from build123d import *

# Parameters (mm, degrees)
BOSS_EXTRUDE1_DEPTH = 24.14


with BuildPart() as part:
    # Sketch3 → Boss-Extrude1 (new body)
    with BuildSketch(Plane.XY):
        with BuildLine():
            Line((6.42, 0), (393.58, 0))
            ThreePointArc((393.58, 0), (402.030182258, -6.090546773), (405.136, 3.852))
            Line((405.136, 3.852), (794.864, 296.148))
            ThreePointArc((794.864, 296.148), (806.090546773, 302.030182258), (793.58, 300))
            Line((793.58, 300), (-393.58, 300))
            ThreePointArc((-393.58, 300), (-406.090546773, 302.030182258), (-394.864, 296.148))
            Line((-394.864, 296.148), (-5.136, 3.852))
            ThreePointArc((-5.136, 3.852), (-2.030182258, -6.090546773), (6.42, 0))
        make_face()
        Polygon((64.373333333, 24.14), (719.533333333, 269.825), (391.953333333, 24.14), align=None, mode=Mode.SUBTRACT)
        Polygon((-327.58, 275.86), (3.90530551, 27.246020868), (666.875916529, 275.86), align=None, mode=Mode.SUBTRACT)
    extrude(amount=BOSS_EXTRUDE1_DEPTH)


solid = part.part
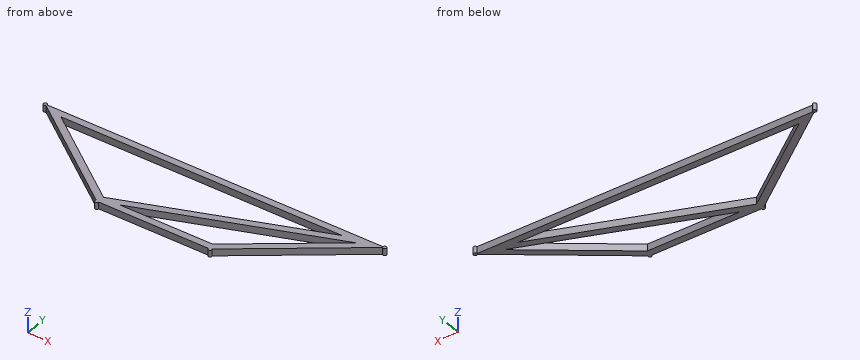
Could you check a few things on this model? Use its own coordinates, in mm. Coordinates: 2 decimals unless noted, no trailing zeros. Order: outer loops, then holes, each group sorted by start corner. A loop starts at its lowest first (then second) coordinate and runs counter-clockwise, first axis right, second up. Notation, with made-up numbers: (40.5, -17.5) - (96.5, -17.5) arc R19 ccw to (96.5, 11.5) - close; hole circle Ø7 at (-19, 65.5). An arc over 180 degrees is marked (long way). Answer in a Markdown table with one row per item. Add a question column.
(1) If we section it at D-D, the plane x = 180.5: Please give me the cut outline in (y, z).
(2) If we section it at B-B, the plane x = -73: Please give me the cut outline in (y, z) (3 decimals), then the cut area to 3 significant figures.
(3) Will these pins go through, and if not, where does the flat tip stop? pin 1 (12 mm diameter, centred on x = 234, z = 16, fed in from -Y); pin 2 (10 mm diameter, centred on x = -86.5, y = 81.5, fed in from -Z); pin 3 (8 mm diameter, centred on y = 264, z = 3, fed in from +X); pin 4 (3 mm diameter, centred on y = 116.5, z = 20, fed in from +X).
(4) If we section it at A-A, the plane z = 15.25: Please give me the cut outline in (x, y) (3 decimals).
(5) If we section it at C-C, the plane y = 206.5: Please give me the cut outline in (x, z).
(6) I need wall thicknesses on L1, parallel to Y at x = 152.5, z = 4.25; L2, parallel to Y at x = 194.5, z = 15.25; L3, parallel to Y at x = -159, z = 8.25 (3 decimals). Which ranges of each line are inside material? Lowest first, please.
Results are:
| question | item | result |
|---|---|---|
| 1 | outline | (0, 0) - (24.14, 0) - (24.14, 24.14) - (0, 24.14) - close; (67.69, 0) - (93.47, 0) - (93.47, 24.14) - (67.69, 24.14) - close; (275.86, 0) - (300, 0) - (300, 24.14) - (275.86, 24.14) - close |
| 2 | outline | (54.75, 0) - (84.925, 0) - (84.925, 24.14) - (54.75, 24.14) - close; (275.86, 0) - (300, 0) - (300, 24.14) - (275.86, 24.14) - close |
| 2 | area | 1,310 mm2 |
| 3 | pin 1 | stops at y = 0 |
| 3 | pin 2 | stops at z = 0 |
| 3 | pin 3 | stops at x = 757.33 |
| 3 | pin 4 | stops at x = 557.33 |
| 4 | outline | (-394.864, 296.148) - (-5.136, 3.852) arc R6.42 ccw (long way) to (6.42, 0) - (393.58, 0) arc R6.42 ccw (long way) to (405.136, 3.852) - (794.864, 296.148) arc R6.42 ccw (long way) to (793.58, 300) - (-393.58, 300) arc R6.42 ccw (long way) to start; hole (-327.58, 275.86) - (3.905, 27.246) - (666.876, 275.86) - close; hole (64.373, 24.14) - (391.953, 24.14) - (719.533, 269.825) - close |
| 5 | outline | (-275.33, 0) - (-235.1, 0) - (-235.1, 24.14) - (-275.33, 24.14) - close; (481.92, 0) - (550.67, 0) - (550.67, 24.14) - (481.92, 24.14) - close; (635.1, 0) - (675.33, 0) - (675.33, 24.14) - (635.1, 24.14) - close |
| 6 | L1 | y = 0 to 24.14, 57.19 to 82.97, 275.86 to 300 |
| 6 | L2 | y = 0 to 24.14, 72.94 to 98.72, 275.86 to 300 |
| 6 | L3 | y = 119.25 to 149.425, 275.86 to 300 |
